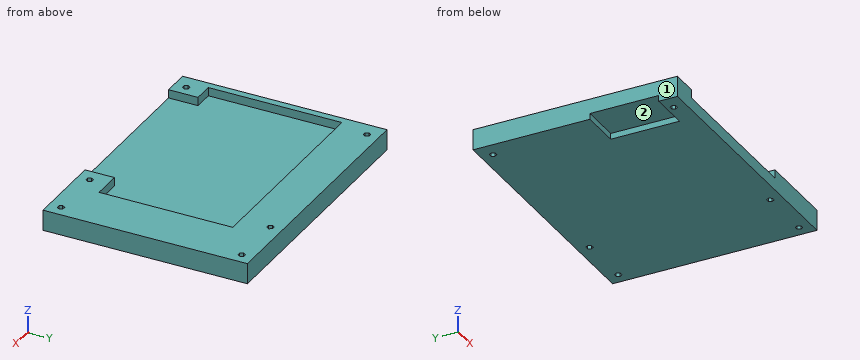
from build123d import *

# Parameters (mm, degrees)
SKETCH_1_W             = 136
SKETCH_1_H             = 104
EXTRUDE_1_DEPTH        = 10.5
SKETCH_1_3_W           = 106.4
SKETCH_1_3_H           = 68
SKETCH_1_3_W_2         = 81.4
SKETCH_1_3_H_2         = 15
CUT_EXTRUDE_1428_DEPTH = 4.3
CUT_EXTRUDE_1767_REACH = 173.529
SKETCH_4_W             = 15
SKETCH_4_H             = 35
SKETCH_4_W_2           = 5.267949192
PCB_DEPTH              = 3


with BuildPart() as part:
    # Sketch 1 → Extrude 1 (new body)
    with BuildSketch(Plane.XY):
        with Locations((68, 52)):
            Rectangle(SKETCH_1_W, SKETCH_1_H)
    extrude(amount=-EXTRUDE_1_DEPTH)

    # Sketch 1_3 → Cut-Extrude 1428 (cut)
    with BuildSketch(Plane.XY):
        with Locations((56.88, 49)):
            Rectangle(SKETCH_1_3_W, SKETCH_1_3_H)
        with Locations((54.38, 7.5)):
            Rectangle(SKETCH_1_3_W_2, SKETCH_1_3_H_2)
    extrude(amount=-CUT_EXTRUDE_1428_DEPTH, mode=Mode.SUBTRACT)

    # Sketch 1_5 → Cut-Extrude 1767 (cut, up to next)
    with BuildSketch(Plane.XY, mode=Mode.PRIVATE) as cut_extrude_1767_sk1:
        Polygon((7.133974596, 96.5), (8.866025404, 96.5), (9.732050808, 98), (8.866025404, 99.5), (7.133974596, 99.5), (6.267949192, 98), align=None)
    cut_extrude_1767_tool1 = extrude(cut_extrude_1767_sk1.sketch, amount=-CUT_EXTRUDE_1767_REACH, mode=Mode.PRIVATE) & part.part
    # Sketch 1_5 → Cut-Extrude 1767 (cut, up to next)
    with BuildSketch(Plane.XY, mode=Mode.PRIVATE) as cut_extrude_1767_sk2:
        Polygon((129.133974596, 96.5), (130.866025404, 96.5), (131.732050808, 98), (130.866025404, 99.5), (129.133974596, 99.5), (128.267949192, 98), align=None)
    cut_extrude_1767_tool2 = extrude(cut_extrude_1767_sk2.sketch, amount=-CUT_EXTRUDE_1767_REACH, mode=Mode.PRIVATE) & part.part
    # Sketch 1_5 → Cut-Extrude 1767 (cut, up to next)
    with BuildSketch(Plane.XY, mode=Mode.PRIVATE) as cut_extrude_1767_sk3:
        Polygon((130.866025404, 7.5), (129.133974596, 7.5), (128.267949192, 6), (129.133974596, 4.5), (130.866025404, 4.5), (131.732050808, 6), align=None)
    cut_extrude_1767_tool3 = extrude(cut_extrude_1767_sk3.sketch, amount=-CUT_EXTRUDE_1767_REACH, mode=Mode.PRIVATE) & part.part
    # Sketch 1_5 → Cut-Extrude 1767 (cut, up to next)
    with BuildSketch(Plane.XY, mode=Mode.PRIVATE) as cut_extrude_1767_sk4:
        Polygon((7.133974596, 4.5), (8.866025404, 4.5), (9.732050808, 6), (8.866025404, 7.5), (7.133974596, 7.5), (6.267949192, 6), align=None)
    cut_extrude_1767_tool4 = extrude(cut_extrude_1767_sk4.sketch, amount=-CUT_EXTRUDE_1767_REACH, mode=Mode.PRIVATE) & part.part
    # Sketch 1_5 → Cut-Extrude 1767 (cut, up to next)
    with BuildSketch(Plane.XY, mode=Mode.PRIVATE) as cut_extrude_1767_sk5:
        Polygon((101.133974596, 4.5), (102.866025404, 4.5), (103.732050808, 6), (102.866025404, 7.5), (101.133974596, 7.5), (100.267949192, 6), align=None)
    cut_extrude_1767_tool5 = extrude(cut_extrude_1767_sk5.sketch, amount=-CUT_EXTRUDE_1767_REACH, mode=Mode.PRIVATE) & part.part
    # Sketch 1_5 → Cut-Extrude 1767 (cut, up to next)
    with BuildSketch(Plane.XY, mode=Mode.PRIVATE) as cut_extrude_1767_sk6:
        Polygon((103.732050808, 98), (102.866025404, 99.5), (101.133974596, 99.5), (100.267949192, 98), (101.133974596, 96.5), (102.866025404, 96.5), align=None)
    cut_extrude_1767_tool6 = extrude(cut_extrude_1767_sk6.sketch, amount=-CUT_EXTRUDE_1767_REACH, mode=Mode.PRIVATE) & part.part
    add(cut_extrude_1767_tool1.solids().sort_by_distance((8, 98, 0))[0], mode=Mode.SUBTRACT)
    add(cut_extrude_1767_tool2.solids().sort_by_distance((130, 98, 0))[0], mode=Mode.SUBTRACT)
    add(cut_extrude_1767_tool3.solids().sort_by_distance((130, 6, 0))[0], mode=Mode.SUBTRACT)
    add(cut_extrude_1767_tool4.solids().sort_by_distance((8, 6, 0))[0], mode=Mode.SUBTRACT)
    add(cut_extrude_1767_tool5.solids().sort_by_distance((102, 6, 0))[0], mode=Mode.SUBTRACT)
    add(cut_extrude_1767_tool6.solids().sort_by_distance((102, 98, 0))[0], mode=Mode.SUBTRACT)

    # Sketch 4 → PCB (cut)
    with BuildSketch(Plane(origin=(0, 0, -10.5), x_dir=(-1, 0, 0), z_dir=(0, 0, -1))):
        with Locations((-12.767949192, 27)):
            Rectangle(SKETCH_4_W, SKETCH_4_H)
        with Locations((-2.633974596, 27)):
            Rectangle(SKETCH_4_W_2, SKETCH_4_H)
    extrude(amount=-PCB_DEPTH, mode=Mode.SUBTRACT)


solid = part.part
Can you work these out from the model? Positions are in its coordinate system, mm. Face numbers are marked on the shaded views. Round coordinates to 2 decimals unless told otherwise and drop trailing zeros. Write each loop counter-clockwise with the first axis right and the second up, starting at its lowest first coordinate (ties: lowest second). Pieces come first, ordered by that corner, then holes. Notation, with made-up numbers: (0, -17.75) -> (57, -17.75) arc R31 cw to (57, 11.25) -> close; hole circle Ø3 at (81, 17). An arc over 180 degrees is marked (long way). One line per question, with ' | ' between items. Start each with the question number.
1) Suppose I cut it at B-B on x = 82.5. Write out the boundary of the cut face in (y, z), then the cut area to 3 significant figures.
2) Suppose I cut it at D-D on x = 97. Write out the boundary of the cut face in (y, z), then the cut area to 3 significant figures.
3) Suppose I cut it at A-A on y = 75. Write out the boundary of the cut face in (x, z), then the cut area to 3 significant figures.
4) If we mould it in two halves opening along Y, with no side actions, what happens to the marked faces 1 and 2? For each: released by +Y, released by -Y, zero draft, split by the parting line, or undercut.
5) I need wall thicknesses on line 1 (X direction, y = 30, z = -2.25); line 2 (Z direction, x = 32.5, y = 65.5); line 3 (Y direction, x = 57, z = -0.25). Which ranges of each line are inside material? Lowest first, please. Write a range as [from, to].
6) Suppose I cut it at C-C on z = -9. Count the separate pieces of the cut face and the enclosed holes in it, then the cut area to 3 significant figures.
7) I'm going to push a flat-ended pin straight in: P1, Ø3.5, axis at y = 27.5, z = -9.5, coming from the -X side. Where does the tip first touch, or does it pass through?
Return value:
1) outline: (0, -10.5) -> (104, -10.5) -> (104, 0) -> (83, 0) -> (83, -4.3) -> (0, -4.3) -> close | area: 735 mm2
2) outline: (0, -10.5) -> (104, -10.5) -> (104, 0) -> (83, 0) -> (83, -4.3) -> (15, -4.3) -> (15, 0) -> (0, 0) -> close | area: 800 mm2
3) outline: (0, -10.5) -> (136, -10.5) -> (136, 0) -> (110.08, 0) -> (110.08, -4.3) -> (3.68, -4.3) -> (3.68, 0) -> (0, 0) -> close | area: 970 mm2
4) face 1: zero draft | face 2: undercut
5) line 1: x = [0, 3.68], [110.08, 136] | line 2: z = [-10.5, -4.3] | line 3: y = [83, 104]
6) separate pieces: 1 | enclosed holes: 6 | area: 13,400 mm2
7) P1: stops at x = 20.27
